Source: CAD feature listing. Evaluate the final solid. Frame: model axes, mm. Face numbers are marked on the shaded views. A direction names the side the tool comes from. Round coordinates to 2 decimals unless told otherwise and drop trailing zeros. Order: outer loops, then holes, each group sorted by start corner. A loop starts at its lowest first (then second) coordinate and runs counter-clockwise, first axis right, second up.
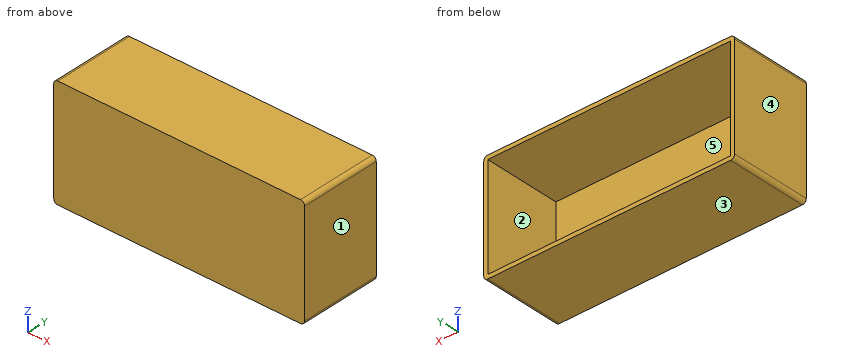
```python
from build123d import *

# Parameters (mm, degrees)
BOSS_EXTRUDE1_DEPTH = 40
SHELL1_START        = 2
SHELL1_OUTLINE_W    = 38
SHELL1_OUTLINE_H    = 51
SHELL1_DEPTH        = 120


# Read off the part's stored shape, not the designer's step: Shell1
with BuildPart() as part:
    # Sketch1 → Boss-Extrude1 (new body)
    with BuildSketch(Plane(origin=(0, 0, 0), x_dir=(1, 0, 0), z_dir=(0, 1, 0))):
        with BuildLine():
            Line((2, 0), (122, 0))
            ThreePointArc((122, 0), (123.414213562, 0.585786438), (124, 2))
            Line((124, 2), (124, 53))
            ThreePointArc((124, 53), (123.414213562, 54.414213562), (122, 55))
            Line((122, 55), (2, 55))
            ThreePointArc((2, 55), (0.585786438, 54.414213562), (0, 53))
            Line((0, 53), (0, 2))
            ThreePointArc((0, 2), (0.585786438, 0.585786438), (2, 0))
        make_face()
    extrude(amount=BOSS_EXTRUDE1_DEPTH)

    # Shell1 outline → Shell1 (cut)
    with BuildSketch(Plane.YZ.offset(SHELL1_START)):
        with Locations((21, -27.5)):
            Rectangle(SHELL1_OUTLINE_W, SHELL1_OUTLINE_H)
    extrude(amount=SHELL1_DEPTH, mode=Mode.SUBTRACT)


solid = part.part
```
1. Access query for the marked faces 4 and 5. Directions: +Z, -Z, +X, -X, +Y, -Y. A direction counts if a zero-diameter tool reaches every point of the face in a straight line with its end or side. Return the directions, or none.
2. Pull-direction query (X, two-part tool) for the marked faces 1, 2 and 3; classes: released by +X, released by -X, zero draft, split by the parting line, or undercut.
3. Section B-B on z = -46. Return loops of the section in (x, y).
4. Section C-C on x = 13. Return loops of the section in (y, z), plus the area to 3 significant figures.
5. Section A-A on y = 23. Return loops of the section in (x, z), plus the area to 3 significant figures.
6. Line query: line 1 along Z through (x, y) = (57.5, 9.5); line 2 along X through (y, z) = (8, -28); line 3 along Y through (x, z) = (20, -45). Output: solid intervals per line, ascending.
Result:
1. face 4: +Z, -Z, -X, +Y, -Y
1. face 5: +Y
2. face 1: released by +X
2. face 2: undercut
2. face 3: zero draft
3. outline: (0, 0) - (124, 0) - (124, 40) - (122, 40) - (122, 2) - (2, 2) - (2, 40) - (0, 40) - close
4. outline: (0, -55) - (40, -55) - (40, -53) - (2, -53) - (2, -2) - (40, -2) - (40, 0) - (0, 0) - close
4. area: 262 mm2
5. outline: (0, -53) arc R2 ccw to (2, -55) - (122, -55) arc R2 ccw to (124, -53) - (124, -2) arc R2 ccw to (122, 0) - (2, 0) arc R2 ccw to (0, -2) - close; hole (2, -53) - (122, -53) - (122, -2) - (2, -2) - close
5. area: 697 mm2
6. line 1: z = -55 to -53, -2 to 0
6. line 2: x = 0 to 2, 122 to 124
6. line 3: y = 0 to 2
